Work out the finished part from the listing and answer in its coordinate system (mm). A direction names the side the tool comes from. Give positions to 0.01 mm unless a question says otherwise; leave off trailing zeros. Order: outer loops, then holes, each group sorted by start corner. A loop starts at its lowest first (then second) coordinate and runs counter-clockwise, first axis right, second up.
```python
from build123d import *

# Parameters (mm, degrees)
SKETCH_1_W          = 60.026557182
SKETCH_1_H          = 33.312327563
EXTRUDE_1_DEPTH     = 2
SKETCH_3_R          = 1.5
SKETCH_3_W          = 22
SKETCH_3_H          = 8
CUT_EXTRUDE_1_DEPTH = 10
FILLET_1_R          = 6


with BuildPart() as part:
    # Эскиз1 → Бобышка-Вытянуть1 (new body)
    with BuildSketch(Plane(origin=(0, 0, 0), x_dir=(1, 0, 0), z_dir=(0, 1, 0))):
        Polygon((-82.5, -31), (-82.5, -21), (-82.5, 31), (-31.5, 31), (31.5, 31), (31.5, -31), align=None)
        with Locations((-8.486721409, -2.656163782)):
            Rectangle(SKETCH_1_W, SKETCH_1_H, mode=Mode.SUBTRACT)
    extrude(amount=EXTRUDE_1_DEPTH)

    # Эскиз3 → Вырез-Вытянуть1 (cut)
    with BuildSketch(Plane.XZ.offset(-2)):
        with Locations(Location((15.9, 23.2, 0), (0, 0, 270))):
            Circle(SKETCH_3_R)
        with Locations(Location((15.9, -17.8, 0), (0, 0, 270))):
            Circle(SKETCH_3_R)
        with Locations(Location((-76.22, 22, 0), (0, 0, 270))):
            Circle(SKETCH_3_R)
        with Locations(Location((-76.22, -21, 0), (0, 0, 270))):
            Circle(SKETCH_3_R)
        with Locations((-8, -23)):
            Rectangle(SKETCH_3_W, SKETCH_3_H)
    extrude(amount=CUT_EXTRUDE_1_DEPTH, mode=Mode.SUBTRACT)

    # Скругление1
    fillet_1_edges = [part.edges().sort_by_distance(p)[0] for p in [
        (-82.5, 1, 31),
        (-82.5, 1, -31),
        (31.5, 1, -31),
        (31.5, 1, 31),
    ]]
    fillet(fillet_1_edges, radius=FILLET_1_R)


solid = part.part
```
1. The part is cut by section B-B (x = 15.9). Write down the section's boundary in (y, z).
Findings below:
outline: (0, -31) - (2, -31) - (2, -19.3) - (0, -19.3) - close; (0, -16.3) - (2, -16.3) - (2, -14) - (0, -14) - close; (0, 19.31) - (2, 19.31) - (2, 21.7) - (0, 21.7) - close; (0, 24.7) - (2, 24.7) - (2, 31) - (0, 31) - close
2. The part is cut by section A-A (x = -32.5). Write down the section's boundary in (y, z), then the cut area to 3 significant figures.
Findings below:
outline: (0, -31) - (2, -31) - (2, -14) - (0, -14) - close; (0, 19.31) - (2, 19.31) - (2, 31) - (0, 31) - close
area: 57.4 mm2
3. The part is cut by section C-C (z = -21). Write down the section's boundary in (x, y).
Findings below:
outline: (-82.5, 0) - (-77.72, 0) - (-77.72, 2) - (-82.5, 2) - close; (-74.72, 0) - (-19, 0) - (-19, 2) - (-74.72, 2) - close; (3, 0) - (31.5, 0) - (31.5, 2) - (3, 2) - close
4. The part is cut by section D-D (y = 1.45). Write down the section's boundary in (x, z), then the cut area to 3 significant figures.
Findings below:
outline: (-82.5, -25) arc R6 ccw to (-76.5, -31) - (25.5, -31) arc R6 ccw to (31.5, -25) - (31.5, 25) arc R6 ccw to (25.5, 31) - (-76.5, 31) arc R6 ccw to (-82.5, 25) - close; hole circle Ø3 at (-76.22, -21); hole circle Ø3 at (-76.22, 22); hole (-38.5, -14) - (21.53, -14) - (21.53, 19.31) - (-38.5, 19.31) - close; hole (-19, -27) - (3, -27) - (3, -19) - (-19, -19) - close; hole circle Ø3 at (15.9, -17.8); hole circle Ø3 at (15.9, 23.2)
area: 4,830 mm2
5. Which of the six approach directions +Z, -Z, +X, -X, +Y, -Y give full straight-line access (tool end or side, diameter ignored) to faces 1 (the face through (-24.7, 2, -14.2)), 2 (the face through (21.527, 1, 3))?
Findings below:
face 1: +Z, -Z, +X, -X, +Y
face 2: +Y, -Y
6. Straight lines are drawn through the part: probe 1 along Z at (x, y) = (-76.22, 1.2); probe 2 along Z at (x, y) = (15.9, 0.45); probe 3 along Z at (x, y) = (-18, 1.55). For each, find the intervals that lie inside material, in ascending order.
Findings below:
probe 1: z = -31 to -22.5, -19.5 to 20.5, 23.5 to 31
probe 2: z = -31 to -19.3, -16.3 to -14, 19.31 to 21.7, 24.7 to 31
probe 3: z = -31 to -27, -19 to -14, 19.31 to 31
7. The mould has two halves that part along X. Classify faces 3 (the face through (3, 1, -23)), 4 (the face through (-80.789, 1.014, 29.196)), 5 (the face through (-24.7, 0, -14.2)), 6 (the face through (29.696, 1.014, 29.289)): pulls with the +X half, pulls with the -X half, needs draft (parallel to the pull), parting line crosses it, or undercut.
Findings below:
face 3: undercut
face 4: pulls with the -X half
face 5: needs draft
face 6: pulls with the +X half
